Autodesk Inventor part; units mm, degrees
ref_plane "YZ Plane" through (0, 0, 0) normal (1, 0, 0) x (0, 1, 0)
ref_plane "XZ Plane" through (0, 0, 0) normal (0, 1, 0) x (-1, 0, 0)
ref_plane "XY Plane" through (0, 0, 0) normal (0, 0, 1) x (1, 0, 0)
sketch "Sketch1" plane through (0, 0, 0) normal (0, 0, 1) x (1, 0, 0)
  circle A0 centre (10.778, 11.3281) radius 10
  point P0 (0, 0)
  dimension "d0" = 20
extrude "Extrusion1" add sketch "Sketch1" along normal mid plane 25
sketch "Sketch2" plane through (10.778, 11.3281, 12.5) normal (0, 0, 1) x (1, 0, 0)
  circle A0 centre (0, 0) radius 2.5
  circle A1 centre (0, 0) radius 4
  point P0 (-10.778, -11.3281)
  dimension "d5" = 5
  dimension "d6" = 8
extrude "Extrusion2" cut sketch "Sketch2" against normal through all contours A0
extrude "Extrusion3" cut sketch "Sketch2" against normal blind 17
properties part number "Shaft Coupler 5mm 8mm"
Check sheet for the modelled part. Datum: model origin and axes. Units: mm. Round coordinates to 2 decimals unless told otherwise and drop trailing zeros. Loops run counter-clockwise (first coordinate to the right, second up) from the corner with the lowest first, then second, coordinate; pieces in that order, holes last. Notation, with made-up numbers: (54, -21) -> (100, -21) arc R20 cw to (100, -6) -> close; hole circle Ø9 at (0.25, 4). An arc over 180 degrees is marked (long way). Answer in a Markdown table with one row per item.
Q1. Release check for a two-part mould opening along X. For faces 1 (the face through (13.4, 10.5, -4.5)), 2 (the face through (2.84, 17.41, -0.18)), 3 (the face through (11, 7, 12.5)), 4 (the face through (14.593, 12.53, 4.119)) record: released by +X, released by -X, zero draft, split by the parting line, or undercut.
Data:
| item | result |
|---|---|
| face 1 | undercut |
| face 2 | split by the parting line |
| face 3 | zero draft |
| face 4 | undercut |
Q2. Thickness scan on L1, parallel to X at y = 11.25, z = -6; L2, parallel to X at y = 11.75, z = -5.25; L3, parallel to Z at x = 11.5, y = 8.25. Record the ranges inside material, lowest first.
Data:
| item | result |
|---|---|
| L1 | x = 0.78 to 8.28, 13.28 to 20.78 |
| L2 | x = 0.79 to 8.31, 13.24 to 20.77 |
| L3 | z = -12.5 to -4.5 |
Q3. Sectioned sample at C-C on z = 5.5. Enter the section's corners in (x, y).
Data:
| item | result |
|---|---|
| outline | circle Ø20 at (10.78, 11.33); hole circle Ø8 at (10.78, 11.33) |
Q4. Sectioned sample at A-A on y = 13.25. Enter the section's corners in (x, z).
Data:
| item | result |
|---|---|
| outline | (0.96, -12.5) -> (9.18, -12.5) -> (9.18, -4.5) -> (7.27, -4.5) -> (7.27, 12.5) -> (0.96, 12.5) -> close; (12.38, -12.5) -> (20.59, -12.5) -> (20.59, 12.5) -> (14.29, 12.5) -> (14.29, -4.5) -> (12.38, -4.5) -> close |
Q5. Sectioned sample at D-D on x = 5.5. Enter the section's corners in (y, z), then the cut area to 3 significant figures.
Data:
| item | result |
|---|---|
| outline | (2.83, -12.5) -> (19.82, -12.5) -> (19.82, 12.5) -> (2.83, 12.5) -> close |
| area | 425 mm^2 |
Q6. Go/stop test with flat-tipped pins: P1, Ø10, axis at x = 18, z = -6.5, coming from the +Y side; P2, Ø2.5, axis at x = 9.5, y = 11, coming from the +Z side; P3, Ø5, axis at x = 6.5, z = 6.5, coming from the +Y side. Record where each tip stops, or that it passes through.
Data:
| item | result |
|---|---|
| P1 | stops at y = 21.08 |
| P2 | stops at z = -4.5 |
| P3 | stops at y = 21.17 |
Q7. Sectioned sample at B-B on x = 11.25. Enter the section's corners in (y, z), then the cut area to 3 significant figures.
Data:
| item | result |
|---|---|
| outline | (1.34, -12.5) -> (8.87, -12.5) -> (8.87, -4.5) -> (7.36, -4.5) -> (7.36, 12.5) -> (1.34, 12.5) -> close; (13.78, -12.5) -> (21.32, -12.5) -> (21.32, 12.5) -> (15.3, 12.5) -> (15.3, -4.5) -> (13.78, -4.5) -> close |
| area | 325 mm^2 |
